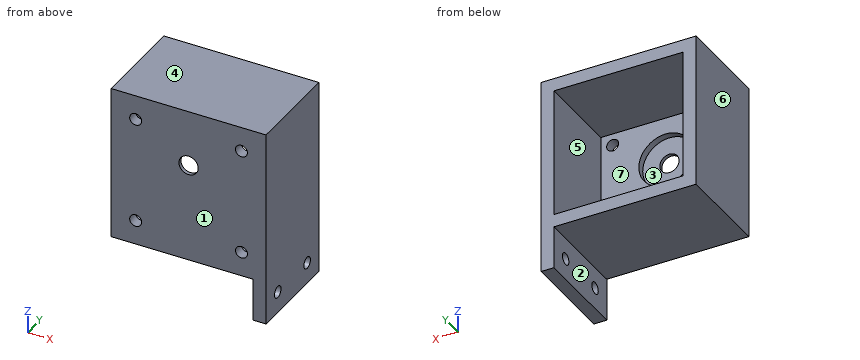
Autodesk Inventor part; units mm, degrees
ref_plane "YZ Plane" through (0, 0, 0) normal (1, 0, 0) x (0, 1, 0)
ref_plane "XZ Plane" through (0, 0, 0) normal (0, 1, 0) x (-1, 0, 0)
ref_plane "XY Plane" through (0, 0, 0) normal (0, 0, 1) x (1, 0, 0)
sketch "Sketch1" plane through (0, 0, 0) normal (0, 1, 0) x (-1, 0, 0)
  line L0 (0, 0) -> (60.5, 0)
  line L1 (60.5, 0) -> (60.5, -60.5)
  line L2 (60.5, -60.5) -> (0, -60.5)
  line L3 (0, -60.5) -> (0, 0)
  line L4 (-6, -66.5) -> (66.5, -66.5)
  line L5 (66.5, -66.5) -> (66.5, 6)
  line L6 (66.5, 6) -> (-6, 6)
  line L7 (-6, 6) -> (-6, -66.5)
  dimension "d0" = 60.5
  dimension "d1" = 60.5
  dimension "d2" = 6
extrude "Extrusion1" add sketch "Sketch1" along normal blind 40
sketch "Sketch2" plane through (0, 0, 0) normal (0, -1, 0) x (1, 0, 0)
  line L0 (-66.5, -60.5) -> (-66.5, 6)
  line L1 (-66.5, 6) -> (6, 6)
  line L2 (6, 6) -> (6, -66.5)
  line L3 (6, -66.5) -> (-66.5, -66.5)
  line L4 (-66.5, -66.5) -> (-66.5, 6)
  point P0 (0, 0)
  point P1 (-63.5, -63.5)
  dimension "d5" = 72.5
  dimension "d6" = 72.5
  dimension "d62" = 6
  dimension "d63" = 6
extrude "Extrusion2" add sketch "Sketch2" along normal blind 5
sketch "Sketch3" plane through (0, -5, 0) normal (0, -1, 0) x (1, 0, 0)
  line L0 (20, -30.25) -> (-80, -30.25) construction
  line L1 (-30.25, 20) -> (-30.25, -80) construction
  circle A0 centre (-55, -5.5) radius 2.8
  circle A1 centre (-5.5, -5.5) radius 2.8
  circle A2 centre (-55, -55) radius 2.8
  circle A3 centre (-5.5, -55) radius 2.8
  point P0 (0, 0)
  dimension "d9" = 100
  dimension "d10" = 30.25
  dimension "d11" = 100
  dimension "d12" = 30.25
  dimension "d13" = 24.75
  dimension "d14" = 24.75
  dimension "d15" = 5.6
  dimension "d18" = 49.5
  dimension "d21" = 49.5
extrude "Extrusion3" cut sketch "Sketch3" against normal blind 5
sketch "Sketch4" plane through (0, 0, 0) normal (0, 1, 0) x (1, 0, 0)
  line L0 (20, 30.25) -> (-80, 30.25) construction
  line L1 (0, 0) -> (-60.5, 0) construction
  line L2 (-30.25, -20) -> (-30.25, 80) construction
  line L3 (0, 60.5) -> (0, 0) construction
  circle A0 centre (-30.25, 20.25) radius 12.5
  dimension "d26" = 100
  dimension "d27" = 30.25
  dimension "d28" = 100
  dimension "d29" = 30.25
  dimension "d30" = 25
  dimension "d31" = 10
extrude "Extrusion4" cut sketch "Sketch4" against normal blind 3.3
sketch "Sketch5" plane through (-30.25, -3.3, -20.25) normal (0, 1, 0) x (1, 0, 0)
  circle A0 centre (0, 0) radius 4.5
  point P0 (30.25, -20.25)
  dimension "d34" = 9
extrude "Extrusion5" cut sketch "Sketch5" against normal blind 2
sketch "Sketch8" plane through (6, 40, -66.5) normal (0, 0, -1) x (-1, 0, 0)
  line L0 (0, 0) -> (72.5, 0)
  line L1 (0, -45) -> (72.5, -45)
  line L2 (0, 0) -> (6, 0)
  line L3 (6, 0) -> (6, -45)
  line L4 (6, -45) -> (0, -45)
  line L5 (0, -45) -> (0, 0)
  point P0 (6, -40)
  dimension "d64" = 6
extrude "Extrusion8" add sketch "Sketch8" along normal blind 20
sketch "Sketch9" plane through (0, -5, -66.5) normal (-1, 0, 0) x (0, 0, 1)
  circle A0 centre (-10, 10) radius 2.75
  line L0 (-20, 0) -> (-20, 45)
  line L1 (0, 0) -> (-20, 0)
  circle A1 centre (-10, 35) radius 2.75
  line L2 (0, 45) -> (-20, 45)
  point P0 (66.5, 5)
  dimension "d67" = 5.5
  dimension "d68" = 10
  dimension "d69" = 10
  dimension "d70" = 5.5
  dimension "d71" = 10
  dimension "d72" = 10
extrude "Extrusion9" cut sketch "Sketch9" against normal blind 6
properties part number "soporte motor"
Can you work these out from the model? Positions are in its coordinate system, mm. Face numbers are marked on the shaded views. A direction names the side the tool comes from. Round coordinates to 2 decimals unless told otherwise and drop trailing zeros. Order: outer loops, then holes, each group sorted by start corner. A loop starts at its lowest first (then second) coordinate and runs counter-clockwise, first axis right, second up. Notation, with made-up numbers: (76, 78.25) -> (95, 78.25) arc R12 ccw to (95, 83.25) -> close; hole circle Ø2 at (-24.5, 10.5). An arc over 180 degrees is marked (long way). Return JSON: item names as keys, results as strings. Group by question number.
1. I need wall thicknesses on line 1 (Y direction, x = 4.8, z = -76.5); line 2 (Z direction, x = -55, y = -3.7); line 3 (Z direction, x = -50, y = 22). Which ranges of each line are inside material? Lowest first, please. Write a range as [from, to].
2. Which directions (+Z, -Z, +X, -X, +Y, -Y) give clear straight access to the entire face, cutting with the end or side of a thin tool? Please do the marked faces 1, 2 and 3.
3. If we section it at A-A, the plane y = 30: Write out the boundary of the cut face in (x, z).
4. Will these pins go through, and if not, where does the flat tip stop? pin 1 (10 mm diameter, centred on x = -6, z = -54.5, fed in from +Y); pin 2 (10 mm diameter, centred on y = 14, z = -75.5, fed in from -X); pin 3 (3.5 mm diameter, centred on x = -55, z = -5.5, fed in from +Y); pin 4 (13.5 mm diameter, centred on x = -31, y = 8, fed in from -Z).
5. We'd pull the mould along Z, two halves only. Please class the marked faces 4, 5, 6 and 7: released by +Z, released by -Z, zero draft, split by the parting line, or undercut.
6. If we section it at B-B, the plane z = -20.25: Write out the boundary of the cut face in (x, y), then the cut area to 3 significant figures.
7. If we section it at D-D, the plane x = -55: Write out the boundary of the cut face in (y, z).
8. If we section it at C-C, the plane x = -30.25: Write out the boundary of the cut face in (y, z), then the cut area to 3 significant figures.
Output values:
{
 "1": {"line 1": "[-5, 2.25], [7.75, 27.25], [32.75, 40]", "line 2": "[-66.5, -57.8], [-52.2, -8.3], [-2.7, 6]", "line 3": "[-66.5, -60.5], [0, 6]"},
 "2": {"face 1": "+Z, -Z, +X, -X, -Y", "face 2": "-Z, -X, +Y, -Y", "face 3": "+Y"},
 "3": {"outline": "(-66.5, -66.5) -> (0, -66.5) -> (0, -73.75) -> (6, -73.75) -> (6, 6) -> (-66.5, 6) -> close; (0, -86.5) -> (6, -86.5) -> (6, -79.25) -> (0, -79.25) -> close; hole (-60.5, -60.5) -> (0, -60.5) -> (0, 0) -> (-60.5, 0) -> close"},
 "4": {"pin 1": "y = 0", "pin 2": "x = 0", "pin 3": "through", "pin 4": "z = -66.5"},
 "5": {"face 4": "released by +Z", "face 5": "undercut", "face 6": "zero draft", "face 7": "undercut"},
 "6": {"outline": "(-66.5, -5) -> (-34.75, -5) -> (-34.75, -3.3) -> (-42.75, -3.3) -> (-42.75, 0) -> (-60.5, 0) -> (-60.5, 40) -> (-66.5, 40) -> close; (-25.75, -5) -> (6, -5) -> (6, 40) -> (0, 40) -> (0, 0) -> (-17.75, 0) -> (-17.75, -3.3) -> (-25.75, -3.3) -> close", "area": "745 mm²"},
 "7": {"outline": "(-5, -66.5) -> (40, -66.5) -> (40, -60.5) -> (0, -60.5) -> (0, -57.8) -> (-5, -57.8) -> close; (-5, -52.2) -> (0, -52.2) -> (0, -8.3) -> (-5, -8.3) -> close; (-5, -2.7) -> (0, -2.7) -> (0, 0) -> (40, 0) -> (40, 6) -> (-5, 6) -> close"},
 "8": {"outline": "(-5, -66.5) -> (40, -66.5) -> (40, -60.5) -> (0, -60.5) -> (0, -32.75) -> (-3.3, -32.75) -> (-3.3, -24.75) -> (-5, -24.75) -> close; (-5, -15.75) -> (-3.3, -15.75) -> (-3.3, -7.75) -> (0, -7.75) -> (0, 0) -> (40, 0) -> (40, 6) -> (-5, 6) -> close", "area": "745 mm²"}
}
